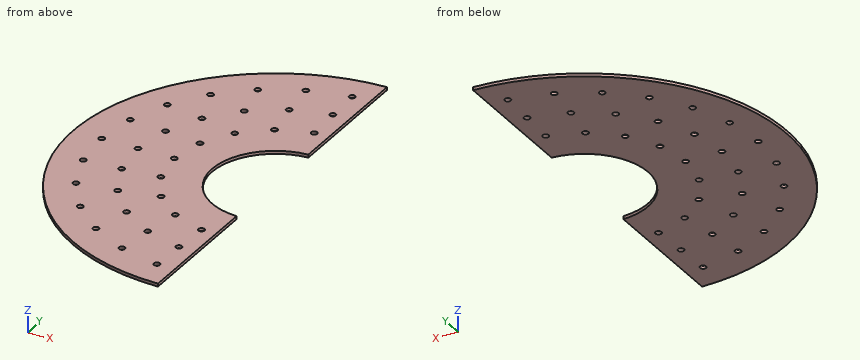
```python
from build123d import *

# Parameters (mm, degrees)
F1_DEPTH  = 6.35
F3_DEPTH  = 6.351
F5_R      = 6.35
F6_DEPTH  = 6.351
F7_R      = 6.35
F8_DEPTH  = 6.351
F9_R      = 6.35
F10_DEPTH = 6.351
F11_W     = 6.35
F11_H     = 938.325346
F12_DEPTH = 6.351


with BuildPart() as f1:
    # F0 (on Top) → F1 (new body)
    with BuildSketch(Plane.XY):
        with BuildLine():
            ThreePointArc((0, 133.35), (94.292689, 94.292689), (133.35, 0))
            ThreePointArc((133.35, 0), (94.292689, -94.292689), (0, -133.35))
            Line((0, -133.35), (0, -425.45))
            ThreePointArc((0, -425.45), (300.83858, -300.83858), (425.45, 0))
            ThreePointArc((425.45, 0), (300.83858, 300.83858), (0, 425.45))
            Line((0, 425.45), (0, 133.35))
        make_face()
        with BuildLine():
            ThreePointArc((0, -133.35), (-133.35, 0), (0, 133.35))
            Line((0, 133.35), (0, 425.45))
            ThreePointArc((0, 425.45), (-425.45, 0), (0, -425.45))
            Line((0, -425.45), (0, -133.35))
        make_face()
    extrude(amount=F1_DEPTH)

    # F2 (on face) → F3 (cut, through all)
    with BuildSketch(Plane.XY.offset(6.35)):
        with BuildLine():
            Line((0, 425.45), (0, 133.35))
            ThreePointArc((0, 133.35), (133.35, 0), (0, -133.35))
            Line((0, -133.35), (0, -425.45))
            ThreePointArc((0, -425.45), (425.45, 0), (0, 425.45))
        make_face()
    extrude(amount=-F3_DEPTH, mode=Mode.SUBTRACT)

    # F5 (on face) → F6 (cut, through all)
    with BuildSketch(Plane.XY.offset(6.35)):
        with Locations((-288.925, 0)):
            Circle(F5_R)
        with Locations((-277.221507, -81.399579)):
            Circle(F5_R)
        with Locations((-243.059177, -156.204648)):
            Circle(F5_R)
        with Locations((-189.205638, -218.354946)):
            Circle(F5_R)
        with Locations((-120.023783, -262.815424)):
            Circle(F5_R)
        with Locations((-41.118315, -285.98416)):
            Circle(F5_R)
        with Locations((41.118315, -285.98416)):
            Circle(F5_R)
        with Locations((120.023783, -262.815424)):
            Circle(F5_R)
        with Locations((189.205638, -218.354946)):
            Circle(F5_R)
        with Locations((243.059177, -156.204648)):
            Circle(F5_R)
        with Locations((277.221507, -81.399579)):
            Circle(F5_R)
        with Locations((288.925, 0)):
            Circle(F5_R)
        with Locations((277.221507, 81.399579)):
            Circle(F5_R)
        with Locations((243.059177, 156.204648)):
            Circle(F5_R)
        with Locations((189.205638, 218.354946)):
            Circle(F5_R)
        with Locations((120.023783, 262.815424)):
            Circle(F5_R)
        with Locations((41.118315, 285.98416)):
            Circle(F5_R)
        with Locations((-41.118315, 285.98416)):
            Circle(F5_R)
        with Locations((-120.023783, 262.815424)):
            Circle(F5_R)
        with Locations((-189.205638, 218.354946)):
            Circle(F5_R)
        with Locations((-243.059177, 156.204648)):
            Circle(F5_R)
        with Locations((-277.221507, 81.399579)):
            Circle(F5_R)
    extrude(amount=-F6_DEPTH, mode=Mode.SUBTRACT)

    # F7 (on face) → F8 (cut, through all)
    with BuildSketch(Plane.XY.offset(6.35)):
        with Locations((-212.725, 0)):
            Circle(F7_R)
        with Locations((-199.896113, -72.756235)):
            Circle(F7_R)
        with Locations((-162.956804, -136.736994)):
            Circle(F7_R)
        with Locations((-106.3625, -184.225254)):
            Circle(F7_R)
        with Locations((-36.939309, -209.493229)):
            Circle(F7_R)
        with Locations((36.939309, -209.493229)):
            Circle(F7_R)
        with Locations((106.3625, -184.225254)):
            Circle(F7_R)
        with Locations((162.956804, -136.736994)):
            Circle(F7_R)
        with Locations((199.896113, -72.756235)):
            Circle(F7_R)
        with Locations((212.725, 0)):
            Circle(F7_R)
        with Locations((199.896113, 72.756235)):
            Circle(F7_R)
        with Locations((162.956804, 136.736994)):
            Circle(F7_R)
        with Locations((106.3625, 184.225254)):
            Circle(F7_R)
        with Locations((36.939309, 209.493229)):
            Circle(F7_R)
        with Locations((-36.939309, 209.493229)):
            Circle(F7_R)
        with Locations((-106.3625, 184.225254)):
            Circle(F7_R)
        with Locations((-162.956804, 136.736994)):
            Circle(F7_R)
        with Locations((-199.896113, 72.756235)):
            Circle(F7_R)
    extrude(amount=-F8_DEPTH, mode=Mode.SUBTRACT)

    # F9 (on face) → F10 (cut, through all)
    with BuildSketch(Plane.XY.offset(6.35)):
        with Locations((-365.125, 0)):
            Circle(F9_R)
        with Locations((-354.515131, -87.380132)):
            Circle(F9_R)
        with Locations((-323.302131, -169.682048)):
            Circle(F9_R)
        with Locations((-273.299987, -242.122661)):
            Circle(F9_R)
        with Locations((-207.414641, -300.491984)):
            Circle(F9_R)
        with Locations((-129.475109, -341.397806)):
            Circle(F9_R)
        with Locations((-44.010955, -362.462828)):
            Circle(F9_R)
        with Locations((44.010955, -362.462828)):
            Circle(F9_R)
        with Locations((129.475109, -341.397806)):
            Circle(F9_R)
        with Locations((207.414641, -300.491984)):
            Circle(F9_R)
        with Locations((273.299987, -242.122661)):
            Circle(F9_R)
        with Locations((323.302131, -169.682048)):
            Circle(F9_R)
        with Locations((354.515131, -87.380132)):
            Circle(F9_R)
        with Locations((365.125, 0)):
            Circle(F9_R)
        with Locations((354.515131, 87.380132)):
            Circle(F9_R)
        with Locations((323.302131, 169.682048)):
            Circle(F9_R)
        with Locations((273.299987, 242.122661)):
            Circle(F9_R)
        with Locations((207.414641, 300.491984)):
            Circle(F9_R)
        with Locations((129.475109, 341.397806)):
            Circle(F9_R)
        with Locations((44.010955, 362.462828)):
            Circle(F9_R)
        with Locations((-44.010955, 362.462828)):
            Circle(F9_R)
        with Locations((-129.475109, 341.397806)):
            Circle(F9_R)
        with Locations((-207.414641, 300.491984)):
            Circle(F9_R)
        with Locations((-273.299987, 242.122661)):
            Circle(F9_R)
        with Locations((-323.302131, 169.682048)):
            Circle(F9_R)
        with Locations((-354.515131, 87.380132)):
            Circle(F9_R)
    extrude(amount=-F10_DEPTH, mode=Mode.SUBTRACT)

    # F11 (on Top) → F12 (cut, through all)
    with BuildSketch(Plane.XY):
        with Locations((-3.175, 4.51836)):
            Rectangle(F11_W, F11_H)
    extrude(amount=F12_DEPTH, mode=Mode.SUBTRACT)


solid = f1.part
```
Geometry check sheet. Reference: the model listing, model coordinates, mm. Coordinates: 2 decimals unless noted, no trailing zeros. Loops run counter-clockwise (first coordinate to the right, second up) from the corner with the lowest first, then second, coordinate; pieces in that order, holes last.
Item 1: Thickness scan on line 1 (Y direction, x = -158, z = 5.75); line 2 (Y direction, x = -195, z = 1); line 3 (Y direction, x = -108.5, z = 5.5). Record the ranges inside material, lowest first.
Item 2: Sectioned sample at D-D, the plane z = 3.5. Count the separate pieces of the cut face and the enclosed holes in it, then the cut area to 3 significant figures.
Item 3: Sectioned sample at A-A, the plane x = -79. Record the boundary of the cut face in (y, z), then the cut area to 3 significant figures.
Item 4: Go/stop test with a flat-tipped pin: pin 1 Ø10 at (x, y) = (-288.925, 0) entering from -Z. Record where the tip stops, or that it passes through.
Item 5: Sectioned sample at C-C, the plane y = -48. Record the boundary of the cut face in (x, z).
Item 6: Sectioned sample at B-B, the plane x = -383.5. Record the boundary of the cut face in (y, z), then the cut area to 3 significant figures.
Check result:
1. line 1: y = -395.02 to -140.71, -132.77 to 132.77, 140.71 to 395.02
1. line 2: y = -378.13 to -220.95, -215.76 to -76.8, -68.71 to 68.71, 76.8 to 215.76, 220.95 to 378.13
1. line 3: y = -411.38 to -190.2, -178.25 to -77.52, 77.52 to 178.25, 190.2 to 411.38
2. separate pieces: 1
2. enclosed holes: 33
2. area: 249,000 mm2
3. outline: (-418.05, 0) - (-107.43, 0) - (-107.43, 6.35) - (-418.05, 6.35) - close; (107.43, 0) - (418.05, 0) - (418.05, 6.35) - (107.43, 6.35) - close
3. area: 3,940 mm2
4. pin 1: passes through
5. outline: (-422.73, 0) - (-124.41, 0) - (-124.41, 6.35) - (-422.73, 6.35) - close
6. outline: (-184.22, 0) - (184.22, 0) - (184.22, 6.35) - (-184.22, 6.35) - close
6. area: 2,340 mm2
